Design review of the part built by this model. Coordinates are the model's own, in mm. A direction names the side the tool comes from. Coordinates: 2 decimals unless noted, no trailing zeros. Order: outer loops, then holes, each group sorted by start corner. A loop starts at its lowest first (then second) coordinate and runs counter-clockwise, first axis right, second up. Notation, with made-up numbers: M -17.5,77 L -13.5,77 A27 cw -13.5,108 Z; hole C 74.25,-19 d11. An arc over 180 degrees is marked long. Answer in a Markdown table with one row per item.
from build123d import *

# Parameters (mm, degrees)
SKETCH_1_W          = 38
SKETCH_1_H          = 38
SKETCH_1_R          = 1
EXTRUDE_1_DEPTH     = 2
CUT_EXTRUDE_1_DEPTH = 27.944387171
EXTRUDE_2_DEPTH     = 9
SKETCH_4_R          = 7.75
EXTRUDE_3_DEPTH     = 16.5


with BuildPart() as part:
    # 草图1 → 凸台-拉伸1 (new body)
    with BuildSketch(Plane(origin=(0, 0, 0), x_dir=(1, 0, 0), z_dir=(0, 1, 0))):
        Rectangle(SKETCH_1_W, SKETCH_1_H)
        with BuildLine():
            ThreePointArc((-8.433484656, 17.913076839), (-7.476946236, 16.95653842), (-8.433484656, 16))
            Line((-8.433484656, 16), (-14, 16))
            ThreePointArc((-14, 16), (-15.414213562, 15.414213562), (-16, 14))
            Line((-16, 14), (-16, 8.433484656))
            ThreePointArc((-16, 8.433484656), (-16.954069804, 7.479414851), (-17.908139609, 8.433484656))
            Line((-17.908139609, 8.433484656), (-17.908139609, 16.166515344))
            ThreePointArc((-17.908139609, 16.166515344), (-17.887296699, 16.3648503), (-17.825678652, 16.554519479))
            ThreePointArc((-17.825678652, 16.554519479), (-18.208704938, 18.205505004), (-16.55600298, 17.829953976))
            ThreePointArc((-16.55600298, 17.829953976), (-16.365644717, 17.892064742), (-16.166515344, 17.913076839))
            Line((-16.166515344, 17.913076839), (-8.433484656, 17.913076839))
        make_face(mode=Mode.SUBTRACT)
        with BuildLine():
            ThreePointArc((-17.908139609, 3.866515344), (-16.954069804, 4.820585149), (-16, 3.866515344))
            Line((-16, 3.866515344), (-16, -3.866515344))
            ThreePointArc((-16, -3.866515344), (-16.954069804, -4.820585149), (-17.908139609, -3.866515344))
            Line((-17.908139609, -3.866515344), (-17.908139609, 3.866515344))
        make_face(mode=Mode.SUBTRACT)
        with BuildLine():
            ThreePointArc((-3.866515344, -17.91801407), (-4.825522379, -16.959007035), (-3.866515344, -16))
            Line((-3.866515344, -16), (3.866515344, -16))
            ThreePointArc((3.866515344, -16), (4.825522379, -16.959007035), (3.866515344, -17.91801407))
            Line((3.866515344, -17.91801407), (-3.866515344, -17.91801407))
        make_face(mode=Mode.SUBTRACT)
        with BuildLine():
            ThreePointArc((17.908139609, -3.866515344), (16.954069804, -4.820585149), (16, -3.866515344))
            Line((16, -3.866515344), (16, 3.866515344))
            ThreePointArc((16, 3.866515344), (16.954069804, 4.820585149), (17.908139609, 3.866515344))
            Line((17.908139609, 3.866515344), (17.908139609, -3.866515344))
        make_face(mode=Mode.SUBTRACT)
        with BuildLine():
            ThreePointArc((3.866515344, 17.91801407), (4.825522379, 16.959007035), (3.866515344, 16))
            Line((3.866515344, 16), (-3.866515344, 16))
            ThreePointArc((-3.866515344, 16), (-4.825522379, 16.959007035), (-3.866515344, 17.91801407))
            Line((-3.866515344, 17.91801407), (3.866515344, 17.91801407))
        make_face(mode=Mode.SUBTRACT)
        with Locations(Location((-14, -14, 0), (0, 0, 270))):
            Circle(SKETCH_1_R, mode=Mode.SUBTRACT)
        with Locations(Location((14, -14, 0), (0, 0, 270))):
            Circle(SKETCH_1_R, mode=Mode.SUBTRACT)
        with Locations(Location((-14, 14, 0), (0, 0, 270))):
            Circle(SKETCH_1_R, mode=Mode.SUBTRACT)
        with Locations(Location((14, 14, 0), (0, 0, 270))):
            Circle(SKETCH_1_R, mode=Mode.SUBTRACT)
    extrude(amount=EXTRUDE_1_DEPTH)

    # 草图2 → 切除-拉伸1 (cut, through all)
    with BuildSketch(Plane(origin=(0, 2, 0), x_dir=(1, 0, 0), z_dir=(0, 1, 0))):
        with BuildLine():
            Line((-17.908139609, -16.166515344), (-17.908139609, -8.433484656))
            ThreePointArc((-17.908139609, -8.433484656), (-16.954069804, -7.479414851), (-16, -8.433484656))
            Line((-16, -8.433484656), (-16, -14))
            ThreePointArc((-16, -14), (-15.414213562, -15.414213562), (-14, -16))
            Line((-14, -16), (-8.433484656, -16.00493723))
            ThreePointArc((-8.433484656, -16.00493723), (-7.48026069, -16.959007035), (-8.433484656, -17.913076839))
            Line((-8.433484656, -17.913076839), (-16.166515344, -17.913076839))
            ThreePointArc((-16.166515344, -17.913076839), (-16.365644717, -17.892064742), (-16.55600298, -17.829953976))
            ThreePointArc((-16.55600298, -17.829953976), (-18.208704938, -18.205505004), (-17.825678652, -16.554519479))
            ThreePointArc((-17.825678652, -16.554519479), (-17.887296699, -16.3648503), (-17.908139609, -16.166515344))
        make_face()
        with BuildLine():
            Line((17.908139609, -16.166515344), (17.908139609, -8.433484656))
            ThreePointArc((17.908139609, -8.433484656), (16.954069804, -7.479414851), (16, -8.433484656))
            Line((16, -8.433484656), (16, -14))
            ThreePointArc((16, -14), (15.414213562, -15.414213562), (14, -16))
            Line((14, -16), (8.433484656, -16.00493723))
            ThreePointArc((8.433484656, -16.00493723), (7.48026069, -16.959007035), (8.433484656, -17.913076839))
            Line((8.433484656, -17.913076839), (16.166515344, -17.913076839))
            ThreePointArc((16.166515344, -17.913076839), (16.365644717, -17.892064742), (16.55600298, -17.829953976))
            ThreePointArc((16.55600298, -17.829953976), (18.208704938, -18.205505004), (17.825678652, -16.554519479))
            ThreePointArc((17.825678652, -16.554519479), (17.887296699, -16.3648503), (17.908139609, -16.166515344))
        make_face()
        with BuildLine():
            Line((8.433484656, 17.913076839), (16.166515344, 17.913076839))
            ThreePointArc((16.166515344, 17.913076839), (16.365644717, 17.892064742), (16.55600298, 17.829953976))
            ThreePointArc((16.55600298, 17.829953976), (18.208704938, 18.205505004), (17.825678652, 16.554519479))
            ThreePointArc((17.825678652, 16.554519479), (17.887296699, 16.3648503), (17.908139609, 16.166515344))
            Line((17.908139609, 16.166515344), (17.908139609, 8.433484656))
            ThreePointArc((17.908139609, 8.433484656), (16.954069804, 7.479414851), (16, 8.433484656))
            Line((16, 8.433484656), (16, 14))
            ThreePointArc((16, 14), (15.414213562, 15.414213562), (14, 16))
            Line((14, 16), (8.433484656, 16.00493723))
            ThreePointArc((8.433484656, 16.00493723), (7.48026069, 16.959007035), (8.433484656, 17.913076839))
        make_face()
        with BuildLine():
            Line((-8.433484656, 17.913076839), (-16.166515344, 17.913076839))
            ThreePointArc((-16.166515344, 17.913076839), (-16.365644717, 17.892064742), (-16.55600298, 17.829953976))
            ThreePointArc((-16.55600298, 17.829953976), (-18.208704938, 18.205505004), (-17.825678652, 16.554519479))
            ThreePointArc((-17.825678652, 16.554519479), (-17.887296699, 16.3648503), (-17.908139609, 16.166515344))
            Line((-17.908139609, 16.166515344), (-17.908139609, 8.433484656))
            ThreePointArc((-17.908139609, 8.433484656), (-16.954069804, 7.479414851), (-16, 8.433484656))
            Line((-16, 8.433484656), (-16, 14))
            ThreePointArc((-16, 14), (-15.414213562, 15.414213562), (-14, 16))
            Line((-14, 16), (-8.433484656, 16.00493723))
            ThreePointArc((-8.433484656, 16.00493723), (-7.48026069, 16.959007035), (-8.433484656, 17.913076839))
        make_face()
    extrude(amount=-CUT_EXTRUDE_1_DEPTH, mode=Mode.SUBTRACT)

    # 草图3 → 凸台-拉伸2 (add)
    with BuildSketch(Plane.XZ):
        with BuildLine():
            Line((-8.5, 2.5), (-9.5, 2.5))
            ThreePointArc((-9.5, 2.5), (-12, 0), (-9.5, -2.5))
            Line((-9.5, -2.5), (-8.5, -2.5))
            Line((-8.5, -2.5), (-8.5, -8.5))
            Line((-8.5, -8.5), (8.5, -8.5))
            Line((8.5, -8.5), (8.5, -2.5))
            Line((8.5, -2.5), (9.5, -2.5))
            ThreePointArc((9.5, -2.5), (12, 0), (9.5, 2.5))
            Line((9.5, 2.5), (8.5, 2.5))
            Line((8.5, 2.5), (8.5, 8.5))
            Line((8.5, 8.5), (-8.5, 8.5))
            Line((-8.5, 8.5), (-8.5, 2.5))
        make_face()
    extrude(amount=EXTRUDE_2_DEPTH)

    # 草图4 → 凸台-拉伸3 (add)
    with BuildSketch(Plane.XZ.offset(9)):
        with Locations(Location((0, 0, 0), (0, 0, 270))):
            Circle(SKETCH_4_R)
    extrude(amount=EXTRUDE_3_DEPTH)


solid = part.part
(1) Add section A-A, the plane z = -11.5. Give the boundary of the cut face in (x, y).
Return value:
| item | result |
|---|---|
| outline | M -19,0 L -17.91,0 L -17.91,2 L -19,2 Z; M -16,0 L 16,0 L 16,2 L -16,2 Z; M 17.91,0 L 19,0 L 19,2 L 17.91,2 Z |
(2) Draft analysis for pull direction X (two halves, no side actions). For faces 1 (the flat face through (0, 0, -9)), 2 (the cylindrical face through (-4.825, 0.986, 16.98)), 3 (the flat face through (8.5, -4, 5)), state which applies: pulls with the +X half, pulls with the -X half, needs draft (parallel to the pull), parting line crosses it, or undercut.
Return value:
| item | result |
|---|---|
| face 1 | needs draft |
| face 2 | undercut |
| face 3 | pulls with the +X half |
(3) Insertion check: pin 1 Ø8 at (x, z) = (-7.5, -7) entering from -Y; pin 2 Ø3 at (y, z) = (-8.5, -3) entering from +X; pin 3 Ø4 at (x, y) = (-3.5, -20.5) entering from +Z; pin 4 Ø8 at (x, y) = (13, -11) entering from -Z. Each pin has a flat end and moves straight along its axis. Give the tip position at first contact, or say it passes through.
Return value:
| item | result |
|---|---|
| pin 1 | stops at y = -25.5 |
| pin 2 | stops at x = 11.5 |
| pin 3 | stops at z = 7.6 |
| pin 4 | stops at z = -2.5 |
(4) Add section D-D, the plane z = 0. Give the boundary of the cut face in (x, y), and give its area (3 significant figures).
Return value:
| item | result |
|---|---|
| outline | M -19,0 L -17.91,0 L -17.91,2 L -19,2 Z; M -16,0 L -12,0 L -12,-9 L -7.75,-9 L -7.75,-25.5 L 7.75,-25.5 L 7.75,-9 L 12,-9 L 12,0 L 16,0 L 16,2 L -16,2 Z; M 17.91,0 L 19,0 L 19,2 L 17.91,2 Z |
| area | 540 mm2 |
(5) Add section C-C, the plane y = -4.75. Give the boundary of the cut face in (x, z), and give its area (3 significant figures).
Return value:
| item | result |
|---|---|
| outline | M -9.5,-2.5 L -8.5,-2.5 L -8.5,-8.5 L 8.5,-8.5 L 8.5,-2.5 L 9.5,-2.5 A2.5 ccw 9.5,2.5 L 8.5,2.5 L 8.5,8.5 L -8.5,8.5 L -8.5,2.5 L -9.5,2.5 A2.5 ccw Z |
| area | 319 mm2 |
(6) For line 1 along X through (y, z) = (1.35, 14); line 2 along Z through (x, y) = (-11, 0.25); line 3 along Z through (x, y) = (-17.5, 1.1), list the stretches that pass through material, from the lowest coordinate up. Write a range as from..to.
Return value:
| item | result |
|---|---|
| line 1 | x = -19..-17.91, -16..-15, -13..13, 15..16, 17.91..19 |
| line 2 | z = -19..-17.91, -16..16, 17.91..19 |
| line 3 | z = -19..-18.5, -7.65..-4.65, 4.65..7.65, 18.5..19 |
(7) Add section B-B, the plane x = 3. Give the boundary of the cut face in (y, z).
Return value:
| item | result |
|---|---|
| outline | M -25.5,-7.15 L -9,-7.15 L -9,-8.5 L 0,-8.5 L 0,-16 L 2,-16 L 2,16 L 0,16 L 0,8.5 L -9,8.5 L -9,7.15 L -25.5,7.15 Z; M 0,-19 L 2,-19 L 2,-17.92 L 0,-17.92 Z; M 0,17.92 L 2,17.92 L 2,19 L 0,19 Z |
(8) For faces 4 (the flat face through (0, 1, 16)), 5 (the flat face through (-8.5, -4, -5)), 6 (the flat face through (-19, 1, 0)), 7 (the flat face through (8.5, -4, -6)), list the 3-axis set-ups (+Z, -Z, +X, -X, +Y, -Y) from which the entire face can be reached by the end or side of a thin tool; tool diameter is ignored.
Return value:
| item | result |
|---|---|
| face 4 | +Y, -Y |
| face 5 | -Z, -X, -Y |
| face 6 | +Z, -Z, -X, +Y, -Y |
| face 7 | -Z, +X, -Y |
